from build123d import *

# Parameters (mm, degrees)
F0_R        = 11.2
F1_DEPTH    = 7
F2_R        = 1.5
F3_T1_DEPTH = 36.7018774228
F3_T4_ANGLE = 72.934456587
F3_T6_ANGLE = 45.7548994245
F3_T8_ANGLE = 56.9956661229


# Not quite as in the source:
# - a fillet or chamfer that OpenCascade refuses, or shapes differently, is made with other operations: its cross-section is extruded or revolved along the edge and cut away or added


with BuildPart() as f1:
    # F0 (on Top) → F1 (new body)
    with BuildSketch(Plane.XY):
        with BuildLine():
            ThreePointArc((-6.1555781478, 35.1188629866), (-15.3560457965, 7.5552379901), (-35.5490386319, -13.3408159018))
            Line((-35.5490386319, -13.3408159018), (-35.5490386319, -22.4113118275))
            ThreePointArc((-35.5490386319, -22.4113118275), (0.6952562714, -16.6112557297), (37.0443966853, -21.713172521))
            Line((37.0443966853, -21.713172521), (37.0443966853, -13.3408159018))
            ThreePointArc((37.0443966853, -13.3408159018), (17.019752647, 8.1099477957), (5.546299275, 35.1188629866))
            Line((5.546299275, 35.1188629866), (-6.1555781478, 35.1188629866))
        make_face()
        Circle(F0_R, mode=Mode.SUBTRACT)
    extrude(amount=F1_DEPTH)

    # F2
    f2_edges = [f1.edges().sort_by_distance(p)[0] for p in [
        (-35.549039, -17.876064, 7),
        (0.695256, -16.611256, 7),
        (-15.356046, 7.555238, 7),
        (17.019753, 8.109948, 7),
        (37.044397, -17.526994, 7),
        (-0.304639, 35.118863, 7),
    ]]
    fillet(f2_edges, radius=F2_R)

    # F3: fillet of radius 5 on 6 edges, made by hand

    # F3_s2 → F3_t1 (cut)
    with BuildSketch(Plane.YZ.offset(-18.6555781478)):
        with BuildLine():
            ThreePointArc((30.1188629866, 0), (33.6543968925, 1.4644660941), (35.1188629866, 5))
            Line((35.1188629866, 5), (35.1188629866, 0))
            Line((35.1188629866, 0), (30.1188629866, 0))
        make_face()
    extrude(amount=F3_T1_DEPTH, mode=Mode.SUBTRACT)

    # F3_s3 → F3_t4 (revolve, cut)
    with BuildSketch(Plane(origin=(-4.3701670653, 47.7604075053, 0), x_dir=(0, 0, 1), z_dir=(-0.0911212144, 0.9958398085, 0))):
        with BuildLine():
            ThreePointArc((0, 3.2563304614), (1.4644660941, -0.2792034445), (5, -1.7436695386))
            Line((5, -1.7436695386), (0, -1.7436695386))
            Line((0, -1.7436695386), (0, 3.2563304614))
        make_face()
    revolve(axis=Axis((-71.5118436224, 41.6168178894, 0), (0, 0, -1)), revolution_arc=F3_T4_ANGLE, mode=Mode.SUBTRACT)

    # F3_s5 → F3_t6 (revolve, cut)
    with BuildSketch(Plane(origin=(-49.5559041376, -21.4739784979, 0), x_dir=(0, 0, 1), z_dir=(-0.9175572913, -0.3976035931, 0))):
        with BuildLine():
            ThreePointArc((0, -0.7975032251), (1.4644660941, -4.333037131), (5, -5.7975032251))
            Line((5, -5.7975032251), (0, -5.7975032251))
            Line((0, -5.7975032251), (0, -0.7975032251))
        make_face()
    revolve(axis=Axis((1.8836501986, -140.182005695, 0), (0, 0, -1)), revolution_arc=F3_T6_ANGLE, mode=Mode.SUBTRACT)

    # F3_s7 → F3_t8 (revolve, cut)
    with BuildSketch(Plane(origin=(45.161339961, -24.4990526211, 0), x_dir=(0, 0, 1), z_dir=(0.8789929725, -0.4768347243, 0))):
        with BuildLine():
            ThreePointArc((5, -5.0138287397), (1.4644660941, -3.5493626456), (0, -0.0138287397))
            Line((0, -0.0138287397), (0, -5.0138287397))
            Line((0, -5.0138287397), (5, -5.0138287397))
        make_face()
    revolve(axis=Axis((87.8129156777, 54.1244901178, 0), (0, 0, -1)), revolution_arc=F3_T8_ANGLE, mode=Mode.SUBTRACT)


solid = f1.part
Source: CAD feature listing. Evaluate the final solid. Frame: model axes, mm. Give positions to 0.01 mm unless a question says otherwise; leave off trailing zeros. Write each loop counter-clockwise with the first axis right and the second up, starting at its lowest first coordinate (ties: lowest second). Pieces come first, ordered by that corner, then holes. Notation, with made-up numbers: (-37, 30) -> (22, 30) arc R15 ccw to (22, 53) -> close; hole circle Ø9 at (38.25, 82.25). An arc over 180 degrees is marked (long way). Return JSON: item names as keys, results as strings. Group by question number.
1. Mould query, pull axis X, two halves, no side actions, for faces 1 (the face through (0.18, -16.617, 5.246)), 2 (the face through (17.25, 7.76, 5.25)), 3 (the face through (-35.549, -18, 3)). Classes: +X half, -X half, draft (parallel to the pull), parting line (faces both ways), or undercut.
2. Pin query (flat end, axial travel): pin 1 Ø12 at (x, y) = (3.5, -16.5) entering from -Z; pin 2 Ø1.5 at (x, z) = (7, 4.5) entering from -Y; pin 3 Ø1 at (x, z) = (26.5, 2.5) entering from -Y. Return the tip coordinate at first contact, or that it passes through.
3. Section A-A, the plane z = 1. Output: boundary loops of the cut face in (x, y), then the cut area to 3 significant figures.
4. Material intervals for line 1 (Y direction, x = 0, z = 5.5); line 2 (X direction, y = 9.5, z = 2.5); line 3 (Y direction, x = 0, z = 3.75), sorted ascending. Write a range as from..to.
Determined:
{
 "1": {"face 1": "undercut", "face 2": "+X half", "face 3": "-X half"},
 "2": {"pin 1": "stops at z = 0", "pin 2": "stops at y = -16.74", "pin 3": "stops at y = -18.68"},
 "3": {"outline": "(-35.55, -20.31) arc R125.58 cw to (37.04, -19.63) -> (37.04, -15.83) arc R86.43 cw to (3.97, 33.12) -> (-4.37, 33.12) arc R67.68 cw to (-35.55, -15.72) -> close; hole circle Ø22.4 at (0, 0)", "area": "1,170 mm2"},
 "4": {"line 1": "y = -16.62..-11.2, 11.2..35.12", "line 2": "x = -13.45..-5.93, 5.93..15.35", "line 3": "y = -16.46..-11.2, 11.2..34.96"}
}
